Geometry: see drawing. Coordinates: mm, zero at the bounding-box minimum. A direction names the side the tool comes from. Give positions to 0.01 mm unless a question says otherwise; leave off trailing zeros. Write each loop counter-clockwise with the first axis right and the second up, starting at its lowest first coordinate (ties: lowest second). Pieces come first, ordered by that corner, then holes. Notation, with made-up numbers: (5.5, 49) -> (23.5, 49) arc R14 ccw to (23.5, 58) -> close; hole circle Ø2 at (22.25, 16.5). An arc over 180 degrees is marked (long way). Use CSV: the item, a comma, the result in double quotes. Start each with the question number.
1) Set-up query: the marked faces 4 and 5. Return all of +Z, -Z, +X, -X, +Y, -Y with unobstructed straight access to the full face (end or side cutting, diameter ignored); none if empty.
2) Section A-A (y = 4.6). Output: boundary loops of the cut face in (x, z) (1 decimal).
3) Draft query along Y for the marked faces 1, 2 and 3. Return one class per face: pulls with the +Y half, pulls with the -Y half, needs draft (parallel to the pull), parting line crosses it, or undercut.
4) Contact query for flat-ended pins moving along their axis: P1, Ø1.5, axis at y = 4.5, z = 1, coming from the -X side; P2, Ø1, axis at x = 3, z = 2.5, coming from the +Y side; P3, Ø2, axis at x = 6, y = 7, coming from the -Z side; P4, Ø2.5, axis at x = 4.6, y = 4.6, coming from the -Z side. Output: stop coordinate, or through.
5) Section C-C (z = 1.75). Output: boundary loops of the cut face in (x, y), plus the area to 3 significant figures.
6) Material intervals for line 1 (Y direction, x = 4.6, z = 2.2); line 2 (Z direction, x = 6, y = 8.5) (1 decimal); line 3 (X direction, y = 4, z = 0.25) (1 decimal), sorted ascending. Write a range as [from, to].
7) Section D-D (x = 2). Output: boundary loops of the cut face in (y, z) (1 decimal), plus the area to 3 significant figures.
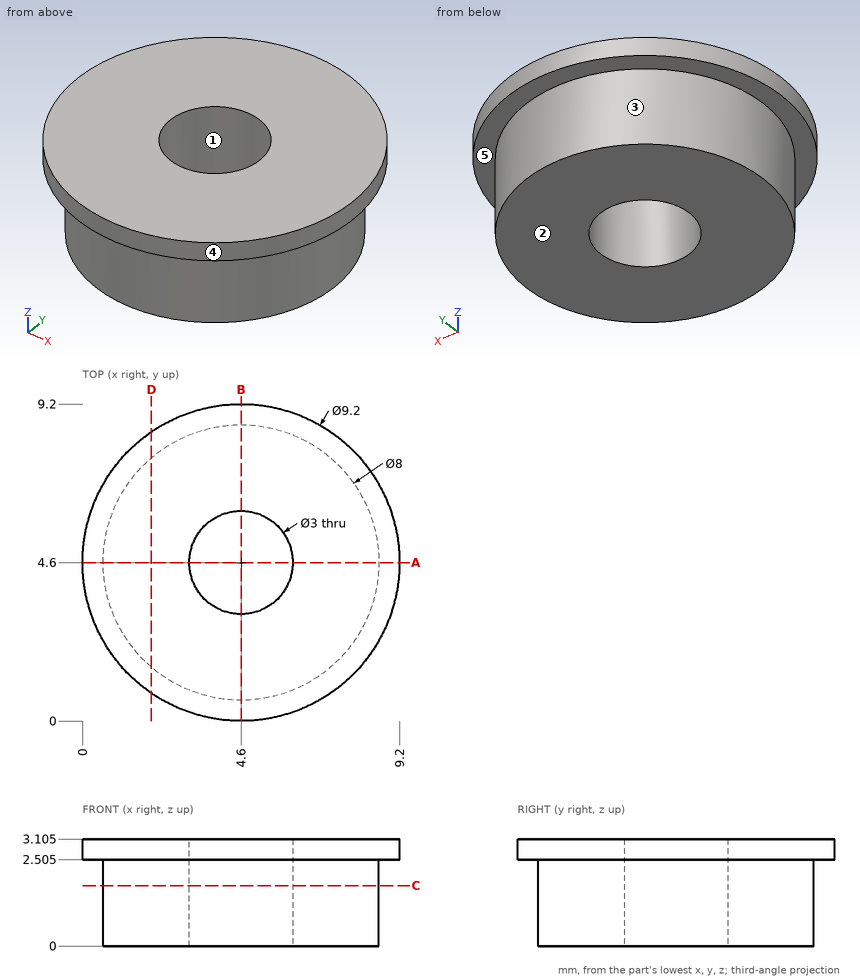
Answers follow:
1,face 4,"+Z, -Z"
1,face 5,"-Z"
2,outline,"(0, 2.5) -> (0.6, 2.5) -> (0.6, 0) -> (3.1, 0) -> (3.1, 3.1) -> (0, 3.1) -> close; (6.1, 0) -> (8.6, 0) -> (8.6, 2.5) -> (9.2, 2.5) -> (9.2, 3.1) -> (6.1, 3.1) -> close"
3,face 1,"undercut"
3,face 2,"needs draft"
3,face 3,"parting line crosses it"
4,P1,"stops at x = 0.6"
4,P2,"stops at y = 9.07"
4,P3,"stops at z = 0"
4,P4,"passes through"
5,outline,"circle Ø8 at (4.6, 4.6); hole circle Ø3 at (4.6, 4.6)"
5,area,"43.2 mm^2"
6,line 1,"y = [0.6, 3.1], [6.1, 8.6]"
6,line 2,"z = [2.5, 3.1]"
6,line 3,"x = [0.6, 3.2], [6, 8.6]"
7,outline,"(0.8, 2.5) -> (1.6, 2.5) -> (1.6, 0) -> (7.6, 0) -> (7.6, 2.5) -> (8.4, 2.5) -> (8.4, 3.1) -> (0.8, 3.1) -> close"
7,area,"19.8 mm^2"
